Work out the finished part from the listing and answer in its coordinate system (mm). A direction names the side the tool comes from. Round coordinates to 2 decimals unless told otherwise and drop trailing zeros. Write each loop counter-clockwise with the first axis right and the second up, starting at its lowest first coordinate (ties: lowest second). Pieces come first, ordered by that corner, then holes.
1. A tool of negligible diameter and unlimited length cuts with its end or side. For faces 3 (the face through (135, -58, -6)), 4 (the face through (150, -1, -1)), 5 (the face through (3, 1, -4)), from which of +Z, -Z, +X, -X, +Y, -Y can it reach the whole face along a straight path? Write none if from no direction.
2. Determine the mould class of faces 1 (the face through (73.331, 58.521, -5.974)), 2 (the face through (99.246, -39.813, -0.986)) for opening direction Y: pulls with the +Y half, pulls with the -Y half, needs draft (parallel to the pull), parting line crosses it, or undercut.
3. Straight lines are drawn through the part: probe 1 along Y at (x, z) = (135, -2.1); probe 2 along Y at (x, z) = (24, -8.75); probe 3 along Y at (x, z) = (15, -1.9). For each, find the intervals that lie inside material, in ascending order.
4. Find section C-C (x = 15). Write down the section's boundary in (y, z), and give its area (3 significant figures).
5. Find section A-A (y = 20). Write down the section's boundary in (x, z).
6. Find section D-D (y = 0). Write down the section's boundary in (x, z).
7. Find section B-B (x = 51.5). Write down the section's boundary in (y, z).
8. Flat-ended cylindrical pins translate along their axes: pin 1 Ø5 at (x, y) = (135, -40) entering from -Z; pin 2 Ø1.5 at (y, z) = (47, -8) entering from +X; pin 3 Ø14.5 at (x, y) = (135, -20) entering from -Z. Find the tip coordinate at first contact, or state that the pin passes through.
```python
from build123d import *

# Parameters (mm, degrees)
COPYSKETCH010_W   = 150
COPYSKETCH010_H   = 120
COPYSKETCH010_R   = 1.75
COPYSKETCH010_R_2 = 4.25
COPYSKETCH010_R_3 = 6.25
COPYSKETCH010_R_4 = 8.25
COPYSKETCH010_W_2 = 15
COPYSKETCH010_H_2 = 15
PAD_DEPTH         = 3
PAD001_DEPTH      = 7
SKETCH001_R       = 1.75
POCKET_DEPTH      = 225.01
SKETCH002_R       = 1.75
POCKET001_DEPTH   = 5.01
SKETCH003_W       = 33
SKETCH003_H       = 20
POCKET002_DEPTH   = 1


with BuildPart() as part:
    # CopySketch010 → Pad (new body)
    with BuildSketch(Plane(origin=(0, 0, 0), x_dir=(-1, 0, 0), z_dir=(0, 0, -1))):
        with Locations((-75, 0)):
            Rectangle(COPYSKETCH010_W, COPYSKETCH010_H)
        with Locations((-146, 56)):
            Circle(COPYSKETCH010_R, mode=Mode.SUBTRACT)
        with Locations((-146, -56)):
            Circle(COPYSKETCH010_R, mode=Mode.SUBTRACT)
        with Locations((-110, -40)):
            Circle(COPYSKETCH010_R_2, mode=Mode.SUBTRACT)
        with Locations((-95, -40)):
            Circle(COPYSKETCH010_R_2, mode=Mode.SUBTRACT)
        with Locations((-51.5, -40)):
            Circle(COPYSKETCH010_R, mode=Mode.SUBTRACT)
        with Locations((-23.5, -40)):
            Circle(COPYSKETCH010_R, mode=Mode.SUBTRACT)
        with Locations((-135, -40)):
            Circle(COPYSKETCH010_R_2, mode=Mode.SUBTRACT)
        with Locations((-135, -20)):
            Circle(COPYSKETCH010_R_3, mode=Mode.SUBTRACT)
        with Locations((-73, -40)):
            Circle(COPYSKETCH010_R_4, mode=Mode.SUBTRACT)
        with Locations((-135, 0)):
            Circle(COPYSKETCH010_R_2, mode=Mode.SUBTRACT)
        with Locations((-135, 20)):
            Circle(COPYSKETCH010_R_3, mode=Mode.SUBTRACT)
        with Locations((-115, 35)):
            Circle(COPYSKETCH010_R, mode=Mode.SUBTRACT)
        with Locations((-115, 15)):
            Circle(COPYSKETCH010_R, mode=Mode.SUBTRACT)
        with Locations((-15, 35)):
            Circle(COPYSKETCH010_R, mode=Mode.SUBTRACT)
        with Locations((-15, 15)):
            Circle(COPYSKETCH010_R, mode=Mode.SUBTRACT)
        with Locations((-37.5, -40)):
            Rectangle(COPYSKETCH010_W_2, COPYSKETCH010_H_2, mode=Mode.SUBTRACT)
    extrude(amount=PAD_DEPTH)

    # Sketch (on DatumPlane) → Pad001 (join)
    with BuildSketch(Plane.XY.offset(-3)):
        Polygon((135, 60), (135, 57), (3, 57), (3, -57), (135, -57), (135, -60), (0, -60), (0, 60), align=None)
    extrude(amount=-PAD001_DEPTH)

    # Sketch001 (on Face6 of Pad001) → Pocket (cut)
    with BuildSketch(Plane(origin=(0, 60, 0), x_dir=(-1, 0, 0), z_dir=(0, 1, 0))):
        with Locations((-25, -6.5)):
            Circle(SKETCH001_R)
        with Locations((-125, -6.5)):
            Circle(SKETCH001_R)
        with Locations((-75, -6.5)):
            Circle(SKETCH001_R)
    extrude(amount=-POCKET_DEPTH, mode=Mode.SUBTRACT)

    # Sketch002 (on Face8 of Pocket) → Pocket001 (cut)
    with BuildSketch(Plane(origin=(0, 0, 0), x_dir=(0, -1, 0), z_dir=(-1, 0, 0))):
        with Locations((50, -6.5)):
            Circle(SKETCH002_R)
        with Locations((-50, -6.5)):
            Circle(SKETCH002_R)
        with Locations((0, -6.5)):
            Circle(SKETCH002_R)
    extrude(amount=-POCKET001_DEPTH, mode=Mode.SUBTRACT)

    # Sketch003 (on Face5 of Pocket001) → Pocket002 (cut)
    with BuildSketch(Plane(origin=(0, 0, -3), x_dir=(1, 0, 0), z_dir=(0, 0, -1))):
        with Locations((102.5, 40)):
            Rectangle(SKETCH003_W, SKETCH003_H)
    extrude(amount=-POCKET002_DEPTH, mode=Mode.SUBTRACT)


solid = part.part
```
Worked answers:
1. face 3: -Z, +X, +Y, -Y
1. face 4: +Z, -Z, +X, +Y, -Y
1. face 5: -Z, +X
2. face 1: needs draft
2. face 2: undercut
3. probe 1: y = -60 to -44.25, -35.75 to -26.25, -13.75 to -4.25, 4.25 to 13.75, 26.25 to 60
3. probe 2: y = -60 to -57, 57 to 60
3. probe 3: y = -60 to 13.25, 16.75 to 33.25, 36.75 to 60
4. outline: (-60, -10) - (-57, -10) - (-57, -3) - (13.25, -3) - (13.25, 0) - (-60, 0) - close; (16.75, -3) - (33.25, -3) - (33.25, 0) - (16.75, 0) - close; (36.75, -3) - (57, -3) - (57, -10) - (60, -10) - (60, 0) - (36.75, 0) - close
4. area: 381 mm2
5. outline: (0, -10) - (3, -10) - (3, -3) - (128.75, -3) - (128.75, 0) - (0, 0) - close; (141.25, -3) - (150, -3) - (150, 0) - (141.25, 0) - close
6. outline: (0, -10) - (3, -10) - (3, -8.25) - (0, -8.25) - close; (0, -4.75) - (3, -4.75) - (3, -3) - (130.75, -3) - (130.75, 0) - (0, 0) - close; (139.25, -3) - (150, -3) - (150, 0) - (139.25, 0) - close
7. outline: (-60, -10) - (-57, -10) - (-57, -3) - (-41.75, -3) - (-41.75, 0) - (-60, 0) - close; (-38.25, -3) - (57, -3) - (57, -10) - (60, -10) - (60, 0) - (-38.25, 0) - close
8. pin 1: passes through
8. pin 2: stops at x = 3
8. pin 3: stops at z = -3
